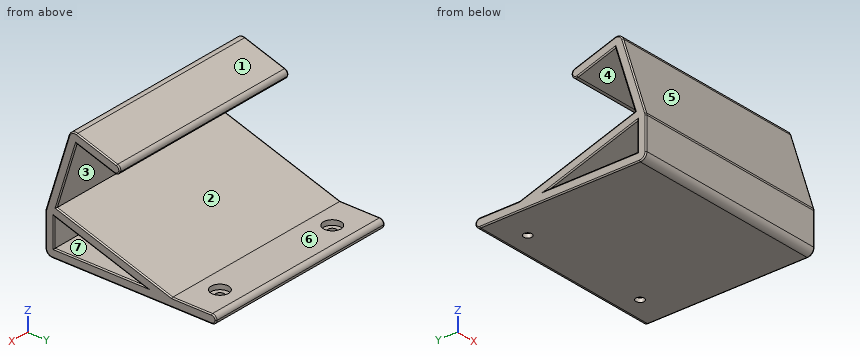
from build123d import *

# Parameters (mm, degrees)
BOSS_EXTRUDE1_DEPTH                                 = 45
CUT_EXTRUDE1_DEPTH                                  = 119.485655068
SKETCH3_W                                           = 90
SKETCH3_H                                           = 97.472123292
BOSS_EXTRUDE2_DEPTH                                 = 4
SKETCH4_W                                           = 17.926774368
SKETCH4_H                                           = 20
CUT_EXTRUDE2_DEPTH                                  = 121.335230998
SKETCH5_W                                           = 90
SKETCH5_H                                           = 17.926774368
BOSS_EXTRUDE3_DEPTH                                 = 4
FILLET7_R                                           = 3
FILLET8_R                                           = 2
FILLET9_R                                           = 0.5
CBORE_FOR_6_BINDING_HEAD_MACHINE_SCREW1_D           = 3.7973
CBORE_FOR_6_BINDING_HEAD_MACHINE_SCREW1_CBORE_D     = 7.9375
CBORE_FOR_6_BINDING_HEAD_MACHINE_SCREW1_CBORE_DEPTH = 2.2098


with BuildPart() as part:
    # Sketch1 → Boss-Extrude1 (new, symmetric)
    with BuildSketch(Plane(origin=(0, 0, 0), x_dir=(0, 0, -1), z_dir=(1, 0, 0))):
        Polygon((-22.597392532, 28.095513), (-28.611508522, 9.021173985), (0, 0), (16.538818973, 52.454432291), (26.538818973, 52.454432291), (55.495428229, -3.170696548), (56.456912684, -5.017691001), (51.947384896, -5.017691001), (24.111559387, 48.454432291), (19.471740318, 48.454432291), (2.612044605, -5.017691001), (-33.629199523, 6.40912938), (-26.412260335, 29.298336198), align=None)
    extrude(amount=BOSS_EXTRUDE1_DEPTH, both=True)

    # Sketch2 → Cut-Extrude1 (cut, through all)
    with BuildSketch(Plane(origin=(45, 0, 0), x_dir=(0, 0, -1), z_dir=(1, 0, 0))):
        Polygon((16.538818973, 52.454432291), (16.538818973, 39.152394197), (19.471740318, 48.454432291), (24.111559387, 48.454432291), (51.947384896, -5.017691001), (56.456912684, -5.017691001), (26.538818973, 52.454432291), align=None)
    extrude(amount=-CUT_EXTRUDE1_DEPTH, mode=Mode.SUBTRACT)

    # Sketch3 → Boss-Extrude2 (add)
    with BuildSketch(Plane(origin=(0, 0, -16.538818973), x_dir=(-1, 0, 0), z_dir=(0, 0, -1))):
        with Locations((0, 23.718370645)):
            Rectangle(SKETCH3_W, SKETCH3_H)
    extrude(amount=BOSS_EXTRUDE2_DEPTH)

    # Sketch4 → Cut-Extrude2 (cut, through all)
    with BuildSketch(Plane.ZY.offset(45)):
        with Locations((-11.575431789, -15.017691001)):
            Rectangle(SKETCH4_W, SKETCH4_H)
    extrude(amount=-CUT_EXTRUDE2_DEPTH, mode=Mode.SUBTRACT)

    # Sketch5 → Boss-Extrude3 (add)
    with BuildSketch(Plane.XZ.offset(5.017691001)):
        with Locations((0, -11.575431789)):
            Rectangle(SKETCH5_W, SKETCH5_H)
    extrude(amount=-BOSS_EXTRUDE3_DEPTH)

    # Fillet7
    fillet7_edges = [part.edges().sort_by_distance(p)[0] for p in [
        (0, -5.017691001, -2.612044605),
        (0, 6.40912938, 33.629199523),
        (0, -5.017691001, -20.538818973),
    ]]
    fillet(fillet7_edges, radius=FILLET7_R)

    # Fillet8
    fillet8_edges = [part.edges().sort_by_distance(p)[0] for p in [
        (0, 72.454432291, -16.538818973),
        (0, 28.095513, 22.597392532),
        (0, 72.454432291, -20.538818973),
        (0, 29.298336198, 26.412260335),
    ]]
    fillet(fillet8_edges, radius=FILLET8_R - 0.0001)  # a hair under: the kernel refuses the full size

    # Fillet9
    fillet9_edges = [part.edges().sort_by_distance(p)[0] for p in [
        (-45, 19.067351598, -16.538818973),
        (-45, 19.067351598, -10.206029367),
        (45, 19.067351598, -10.206029367),
        (-45, -1.017691001, -10.206029367),
        (45, -1.017691001, -10.206029367),
        (-45, 34.218420645, -20.538818973),
        (-45, -5.017691001, -10.30630387),
        (-45, 0.314085064, 14.298188651),
        (-45, 6.982916994, 32.526963772),
        (-45, -4.982775532, -2.61741861),
        (-45, 17.604674228, 25.905141292),
        (-45, -4.139011345, -19.660139316),
        (45, -5.017691001, -10.30630387),
        (45, 0.314085064, 14.298188651),
        (45, 6.982916994, 32.526963772),
        (-45, 4.510586993, 14.305754261),
        (45, -4.982775532, -2.61741861),
        (45, -4.139011345, -19.660139316),
        (-45, 26.227216146, -8.269409486),
        (45, 34.218420645, -20.538818973),
        (45, 61.454482291, -16.538818973),
        (45, 18.33063895, 29.870361994),
        (45, 28.563549105, 26.029754386),
        (45, 27.71300705, 23.332179625),
        (45, 71.868675143, -19.953061824),
        (45, 71.868675143, -17.124576121),
        (-45, 18.33063895, 29.870361994),
        (-45, 28.563549105, 26.029754386),
        (-45, 27.71300705, 23.332179625),
        (-45, 71.868675143, -19.953061824),
        (-45, 71.868675143, -17.124576121),
        (45, 26.227216146, -8.269409486),
        (45, 4.510586993, 14.305754261),
        (45, 17.604674228, 25.905141292),
        (-45, 61.454482291, -16.538818973),
        (45, 19.067351598, -16.538818973),
    ]]
    fillet(fillet9_edges, radius=FILLET9_R)

    # CBORE for #6 Binding Head Machine Screw1 (through all)
    with Locations(Plane.XY.offset(-16.538818973)):
        with Locations((-30, 61.454432291), (30, 61.454432291)):
            CounterBoreHole(CBORE_FOR_6_BINDING_HEAD_MACHINE_SCREW1_D / 2, CBORE_FOR_6_BINDING_HEAD_MACHINE_SCREW1_CBORE_D / 2, CBORE_FOR_6_BINDING_HEAD_MACHINE_SCREW1_CBORE_DEPTH)


solid = part.part
Here's how the part is built. I have some questions about the finished solid (model axes, mm). Face numbers are marked on the shaded views. A direction names the side the tool comes from. Give positions to 0.01 mm unless a question says otherwise; leave off trailing zeros. Order: outer loops, then holes, each group sorted by start corner. A loop starts at its lowest first (then second) coordinate and runs counter-clockwise, first axis right, second up. Notation, with made-up numbers: M 85.5,-29.5 L 124.5,-29.5 A28 cw 124.5,6.5 Z; hole C -5.75,56.25 d9. An arc over 180 degrees is marked long. Answer as a JSON object with one key per item and string values. Group by question number.
1) Suppose I cut it at A-A, the plane x = -30. Count the separate pieces of the cut face and the enclosed holes in it, plus the area to 3 significant figures.
2) Please list where these lines run through material, in increasing order: L1, parallel to Z at x = -5, y = 20; L2, parallel to Z at x = -27.5, y = 21.5; L3, parallel to Y at x = -30, z = -19. Write a range as [from, to].
3) Suppose I cut it at B-B, the plane y = 55. Write out the boundary of the cut face in (x, z), plus the area to 3 significant figures.
4) I'm going to push flat-ended pins straight in: pin 1 Ø4 at (x, z) = (15.5, 21) entering from -Y; pin 2 Ø4 at (x, y) = (8.5, 47.5) entering from +Z; pin 3 Ø3.5 at (x, y) = (30, 61.45) entering from +Z; pin 4 Ø3 at (x, y) = (27.5, 28.5) entering from +Z. Where does each tip first touch, or does it pass through?
5) On a 3-axis mill with a long thin cutter (end or side, diameter ignored), from which of +Z, -Z, +X, -X, +Y, -Y can I reach the whole of each face in a straight line? I mean the marked faces 1, 2 and 3. Say none if no direction works.
6) We'd pull the mould along Y, two halves only. Please class the marked faces 4, 5, 6 and 7: pulls with the +Y half, pulls with the -Y half, needs draft (parallel to the pull), parting line crosses it, or undercut.
Results found:
{
 "1": {"separate pieces": "2", "enclosed holes": "1", "area": "758 mm²"},
 "2": {"L1": "[-20.54, -16.54], [-10.5, -6.31], [25.15, 29.34]", "L2": "[-20.54, -16.54], [-10.97, -6.78], [24.68, 28.87]", "L3": "[-4.64, 59.56], [63.35, 72.4]"},
 "3": {"outline": "M -45,-20.04 A0.5 ccw -44.5,-20.54 L 44.5,-20.54 A0.5 ccw 45,-20.04 L 45,-17.04 A0.5 ccw 44.5,-16.54 L -44.5,-16.54 A0.5 ccw -45,-17.04 Z", "area": "360 mm²"},
 "4": {"pin 1": "y = 1.8", "pin 2": "z = -14.35", "pin 3": "through", "pin 4": "z = 27.14"},
 "5": {"face 1": "+Z, +X, -X, +Y", "face 2": "+X, -X, +Y", "face 3": "+X, -X"},
 "6": {"face 4": "undercut", "face 5": "pulls with the -Y half", "face 6": "needs draft", "face 7": "undercut"}
}
